Could you check a few things on this model? Use its own coordinates, in mm. A direction names the side the tool comes from. Coordinates: 2 decimals unless noted, no trailing zeros. Loops run counter-clockwise (first coordinate to the right, second up) from the corner with the lowest first, then second, coordinate; pieces in that order, holes last.
1) Imagine slicing it at C-C on z = 100. Please give me the cut outline in (x, y), plus the area to 3 significant figures.
2) For faces 1 (the face through (0, 23, 214)), 2 (the face through (0, 25, 217)), 3 (the face through (11.51, -0.98, 145.61)), which set-ups out of +Z, -Z, +X, -X, +Y, -Y let a thin tool reach every point of the face, with its end or its side?
3) Thinking about a two-plate mould opening in X: for faces 4 (the face through (-12.5, 0, 217)), 5 (the face through (10.5, 0, 214)), 6 (the face through (-1.72, -23.99, 374.16)), 7 (the face through (11.51, -0.59, 104.46)), which applies, released by +X, released by -X, zero draft, split by the parting line, or undercut?
4) Will these pins go through, and if not, where does the flat tip stop? P1, Ø5.5, axis at y = 0, z = 150, coming from the +X side; P2, Ø10, axis at x = 1.5, y = -19, coming from the +Z side.
5) Imagine slicing it at A-A on y = -9. Please give me the cut outline in (x, z), plus the area to 3 significant figures.
6) Imagine slicing it at B-B on z = 295. Please give me the cut outline in (x, y), plus the area to 3 significant figures.
7) If I drill on line 1 along X through (y, z) = (11.5, 347); line 2 along Y through (x, z) = (7.75, 392); line 3 along Z through (x, y) = (11.5, 0), over which ranges is the centre line in solid material (lowest first)?
```python
from build123d import *

# Parameters (mm, degrees)
SKETCH_1_W          = 25
SKETCH_1_H          = 50
SKETCH_1_W_2        = 21
SKETCH_1_H_2        = 46
EXTRUDE_1_DEPTH     = 440
SKETCH_2_R          = 12.5
SKETCH_2_R_2        = 4.5
CUT_EXTRUDE_1_DEPTH = 50
SKETCH_3_R          = 4.5
CUT_EXTRUDE_2_DEPTH = 2


with BuildPart() as part:
    # Эскиз1 → Бобышка-Вытянуть1 (new body)
    with BuildSketch(Plane.XY):
        Rectangle(SKETCH_1_W, SKETCH_1_H)
        Rectangle(SKETCH_1_W_2, SKETCH_1_H_2, mode=Mode.SUBTRACT)
    extrude(amount=EXTRUDE_1_DEPTH)

    # Эскиз2 → Вырез-Вытянуть1 (cut)
    with BuildSketch(Plane(origin=(0, 25, 0), x_dir=(1, 0, 0), z_dir=(0, 1, 0))):
        with Locations((0, -440)):
            Circle(SKETCH_2_R)
        with Locations(Location((0, -370, 0), (0, 0, 270))):  # turned: the seam where the file's is
            Circle(SKETCH_2_R_2)
        with Locations(Location((0, -295, 0), (0, 0, 270))):  # turned: the seam where the file's is
            Circle(SKETCH_2_R_2)
    extrude(amount=-CUT_EXTRUDE_1_DEPTH, mode=Mode.SUBTRACT)

    # Эскиз3 → Вырез-Вытянуть2 (cut)
    with BuildSketch(Plane(origin=(12.5, 0, 0), x_dir=(0, 0, -1), z_dir=(1, 0, 0))):
        with Locations(Location((-50, 0, 0), (0, 0, 90))):  # turned: the seam where the file's is
            Circle(SKETCH_3_R)
        with Locations(Location((-100, 0, 0), (0, 0, 90))):  # turned: the seam where the file's is
            Circle(SKETCH_3_R)
        with Locations(Location((-150, 0, 0), (0, 0, 90))):  # turned: the seam where the file's is
            Circle(SKETCH_3_R)
        with Locations(Location((-200, 0, 0), (0, 0, 90))):  # turned: the seam where the file's is
            Circle(SKETCH_3_R)
        with Locations(Location((-250, 0, 0), (0, 0, 90))):  # turned: the seam where the file's is
            Circle(SKETCH_3_R)
    extrude(amount=-CUT_EXTRUDE_2_DEPTH, mode=Mode.SUBTRACT)


solid = part.part
```
Filled in:
1. outline: (-12.5, -25) - (12.5, -25) - (12.5, -4.5) - (10.5, -4.5) - (10.5, -23) - (-10.5, -23) - (-10.5, 23) - (10.5, 23) - (10.5, 4.5) - (12.5, 4.5) - (12.5, 25) - (-12.5, 25) - close
1. area: 266 mm2
2. face 1: +Z, -Z
2. face 2: +Z, -Z, +X, -X, +Y
2. face 3: +X
3. face 4: released by -X
3. face 5: undercut
3. face 6: undercut
3. face 7: zero draft
4. P1: stops at x = -10.5
4. P2: stops at z = 428.34
5. outline: (-12.5, 0) - (-10.5, 0) - (-10.5, 433.22) arc R12.5 cw to (-12.5, 440) - close; (10.5, 0) - (12.5, 0) - (12.5, 440) arc R12.5 cw to (10.5, 433.22) - close
5. area: 1,740 mm2
6. outline: (-12.5, -25) - (-4.5, -25) - (-4.5, -23) - (-10.5, -23) - (-10.5, 23) - (-4.5, 23) - (-4.5, 25) - (-12.5, 25) - close; (4.5, -25) - (12.5, -25) - (12.5, 25) - (4.5, 25) - (4.5, 23) - (10.5, 23) - (10.5, -23) - (4.5, -23) - close
6. area: 248 mm2
7. line 1: x = -12.5 to -10.5, 10.5 to 12.5
7. line 2: y = -25 to -23, 23 to 25
7. line 3: z = 0 to 45.5, 54.5 to 95.5, 104.5 to 145.5, 154.5 to 195.5, 204.5 to 245.5, 254.5 to 435.1
